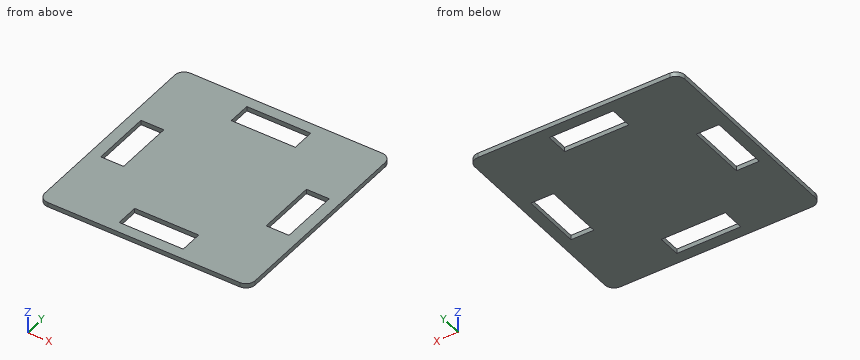
```python
from build123d import *

# Parameters (mm, degrees)
F0_W     = 31.75
F0_H     = 82.55
F0_W_2   = 88.9
F0_H_2   = 31.75
F1_DEPTH = 6.35


with BuildPart() as f1:
    # F0 (on Top) → F1 (new body)
    with BuildSketch(Plane.XY):
        with BuildLine():
            ThreePointArc((-146.05, -124.442522), (-142.330256, -133.422778), (-133.35, -137.142522))
            Line((-133.35, -137.142522), (133.35, -137.142522))
            ThreePointArc((133.35, -137.142522), (142.330256, -133.422778), (146.05, -124.442522))
            Line((146.05, -124.442522), (146.05, 142.257478))
            ThreePointArc((146.05, 142.257478), (142.330256, 151.237734), (133.35, 154.957478))
            Line((133.35, 154.957478), (-133.35, 154.957478))
            ThreePointArc((-133.35, 154.957478), (-142.330256, 151.237734), (-146.05, 142.257478))
            Line((-146.05, 142.257478), (-146.05, -124.442522))
        make_face()
        with Locations((-114.935, 8.907478)):
            Rectangle(F0_W, F0_H, mode=Mode.SUBTRACT)
        with Locations((0, -106.027522)):
            Rectangle(F0_W_2, F0_H_2, mode=Mode.SUBTRACT)
        with Locations((114.935, 8.907478)):
            Rectangle(F0_W, F0_H, mode=Mode.SUBTRACT)
        with Locations((0, 123.842478)):
            Rectangle(F0_W_2, F0_H_2, mode=Mode.SUBTRACT)
    extrude(amount=F1_DEPTH)


solid = f1.part
```
Design review of the part built by this model. Coordinates are the model's own, in mm. Give positions to 0.01 mm unless a question says otherwise; leave off trailing zeros. Order: outer loops, then holes, each group sorted by start corner. A loop starts at its lowest first (then second) coordinate and runs counter-clockwise, first axis right, second up. Notation, with made-up numbers: (85, 22) -> (103, 22) arc R10 cw to (103, 32) -> close; hole circle Ø5 at (-29, -5). An arc over 180 degrees is marked (long way). Write each question's results on one line, items separated by ' | '. Start each with the question number.
Q1. Wall thickness on L1, parallel to X at y = 22.5, z = 6.25; L2, parallel to Y at x = 13, z = 4; L3, parallel to X at y = 117, z = 0.5: over which ranges is each line inside the solid? List them lowest first. Write a range as from..to.
Q2. For pin 1 (6 mm diameter, centred on x = -36, y = 112.5, fed in from +Z), flat-tipped, find the tip position at first contact; note if it passes through.
Q3. Add section A-A on y = 33. Give the boundary of the cut face in (x, z), and give its area (3 significant figures).
Q4. Add section D-D on z = 4. Give the boundary of the cut face in (x, y), and give its area (3 significant figures).
Q5. Add section C-C on x = -113.5. Give the boundary of the cut face in (y, z).
Q6. Add section B-B on x = -5. Give the boundary of the cut face in (y, z), and give its area (3 significant figures).
Found:
1) L1: x = -146.05..-130.81, -99.06..99.06, 130.81..146.05 | L2: y = -137.14..-121.9, -90.15..107.97, 139.72..154.96 | L3: x = -146.05..-44.45, 44.45..146.05
2) pin 1: passes through
3) outline: (-146.05, 0) -> (-130.81, 0) -> (-130.81, 6.35) -> (-146.05, 6.35) -> close; (-99.06, 0) -> (99.06, 0) -> (99.06, 6.35) -> (-99.06, 6.35) -> close; (130.81, 0) -> (146.05, 0) -> (146.05, 6.35) -> (130.81, 6.35) -> close | area: 1,450 mm2
4) outline: (-146.05, -124.44) arc R12.7 ccw to (-133.35, -137.14) -> (133.35, -137.14) arc R12.7 ccw to (146.05, -124.44) -> (146.05, 142.26) arc R12.7 ccw to (133.35, 154.96) -> (-133.35, 154.96) arc R12.7 ccw to (-146.05, 142.26) -> close; hole (-130.81, -32.37) -> (-99.06, -32.37) -> (-99.06, 50.18) -> (-130.81, 50.18) -> close; hole (-44.45, -121.9) -> (44.45, -121.9) -> (44.45, -90.15) -> (-44.45, -90.15) -> close; hole (-44.45, 107.97) -> (44.45, 107.97) -> (44.45, 139.72) -> (-44.45, 139.72) -> close; hole (99.06, -32.37) -> (130.81, -32.37) -> (130.81, 50.18) -> (99.06, 50.18) -> close | area: 74,300 mm2
5) outline: (-137.14, 0) -> (-32.37, 0) -> (-32.37, 6.35) -> (-137.14, 6.35) -> close; (50.18, 0) -> (154.96, 0) -> (154.96, 6.35) -> (50.18, 6.35) -> close
6) outline: (-137.14, 0) -> (-121.9, 0) -> (-121.9, 6.35) -> (-137.14, 6.35) -> close; (-90.15, 0) -> (107.97, 0) -> (107.97, 6.35) -> (-90.15, 6.35) -> close; (139.72, 0) -> (154.96, 0) -> (154.96, 6.35) -> (139.72, 6.35) -> close | area: 1,450 mm2
